Verification items for this drawing (mm, ordinates from the low corner). A direction names the side the tool comes from. Round coordinates to 2 decimals unless told otherwise and drop trailing zeros. Write each loop counter-clockwise with the first axis right and the second up, starting at its lowest first coordinate (ties: lowest second). Pieces come first, ordered by that corner, then holes. Notation, with made-up numbers: (77, 56.5) - (128, 56.5) arc R18 cw to (128, 83.5) - close; hole circle Ø7 at (28.5, 88). An arc over 180 degrees is marked (long way). One line per question, with ' | ' between items. Start each with the question number.
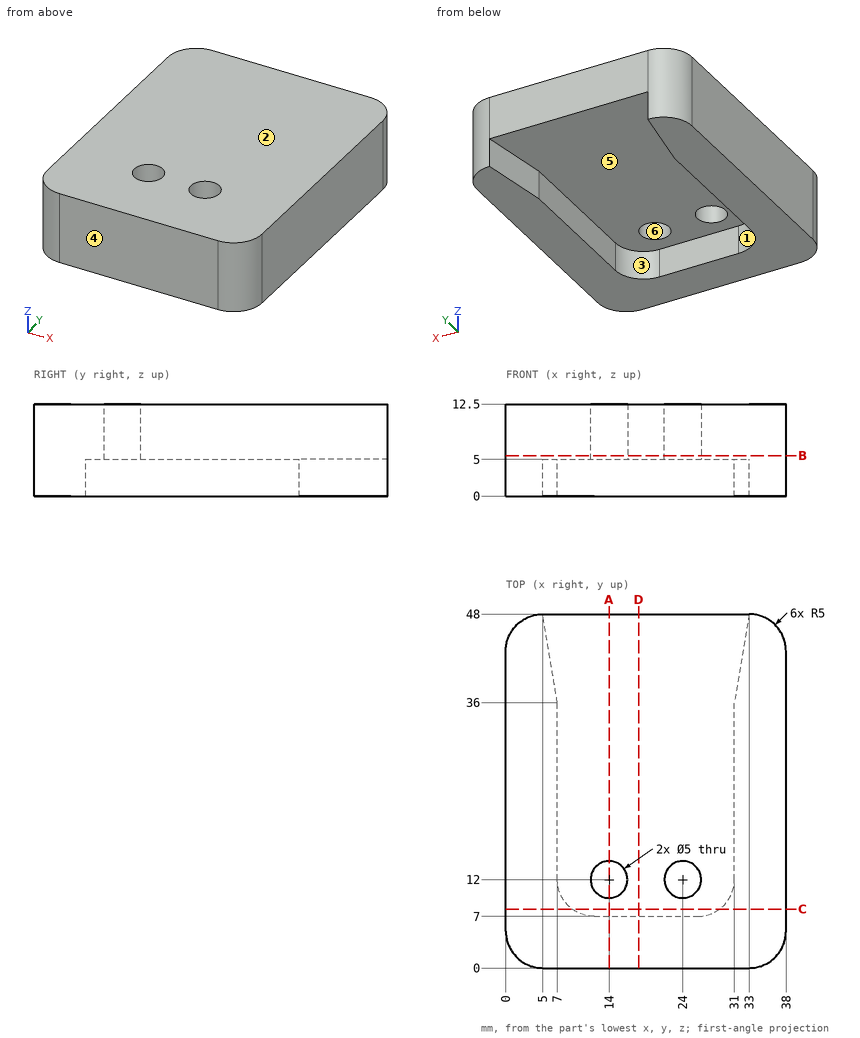
Q1. Section check A-A, the plane x = 14. Record the cut outline in (y, z).
Q2. Draft check along Y on the marked faces 3, 4, 5 and 6. Enter one of: pulls with the +Y half, pulls with the -Y half, needs draft (parallel to the pull), parting line crosses it, or undercut.
Q3. Section check B-B, the plane z = 5.5. Record the cut outline in (x, y).
Q4. Go/stop test with flat-tipped pins: P1, Ø2.5, axis at x = 18, z = 2.5, coming from the +Y side; P2, Ø14, axis at x = 15.5, y = 35, coming from the -Z side. Record where each tip stops, or that it passes through.
Q5. Section check D-D, the plane x = 18. Record the cut outline in (y, z), then the cut area to 3 significant figures.
Q6. Section check C-C, the plane y = 8. Record the cut outline in (x, z).
Q7. Thickness scan on line 1 (Y direction, x = 24, z = 9.5); line 2 (X direction, y = 18, z = 4.5); line 3 (Y direction, x = 21.5, z = 4.5). Record the ranges inside material, lowest first.
Q8. Set-up check for the marked faces 1 and 2: record each of +Z, -Z, +X, -X, +Y, -Y from which the full face is reachable in a straight line by a thin tool's end or side.
Result sheet:
1) outline: (0, 0) - (7, 0) - (7, 5) - (9.5, 5) - (9.5, 12.5) - (0, 12.5) - close; (14.5, 5) - (48, 5) - (48, 12.5) - (14.5, 12.5) - close
2) face 3: pulls with the +Y half | face 4: pulls with the -Y half | face 5: needs draft | face 6: undercut
3) outline: (0, 5) arc R5 ccw to (5, 0) - (33, 0) arc R5 ccw to (38, 5) - (38, 43) arc R5 ccw to (33, 48) - (5, 48) arc R5 ccw to (0, 43) - close; hole circle Ø5 at (14, 12); hole circle Ø5 at (24, 12)
4) P1: y = 7 | P2: z = 5
5) outline: (0, 0) - (7, 0) - (7, 5) - (48, 5) - (48, 12.5) - (0, 12.5) - close | area: 395 mm²
6) outline: (0, 0) - (9, 0) - (9, 5) - (29, 5) - (29, 0) - (38, 0) - (38, 12.5) - (0, 12.5) - close
7) line 1: 0 to 9.5, 14.5 to 48 | line 2: 0 to 7, 31 to 38 | line 3: 0 to 7
8) face 1: -Z, +Y | face 2: +Z, +X, -X, +Y, -Y
